```python
from build123d import *

# Parameters (mm, degrees)
F1_DEPTH = 40
F2_DEPTH = 5
F4_T     = -2
F3_R     = 35.75
F5_DEPTH = 5
F6_D     = 4.5
F6_DEPTH = 2
F6_TIP   = 1.3519363928
F8_DEPTH = 1.5


with BuildPart() as f1:
    # F0 (on Front) → F1 (new body, symmetric)
    with BuildSketch(Plane.XZ):
        Polygon((0, 69.2820323028), (-40, 0), (0, 0), align=None)
    extrude(amount=F1_DEPTH, both=True)

    # F2 (add): a face of the model
    f2_faces = [f1.faces().sort_by_distance(p)[0] for p in [
        (-20, 0, 34.6410161514),
    ]]
    extrude(f2_faces, amount=F2_DEPTH)

    # F4
    f4_openings = [f1.faces().sort_by_distance(p)[0] for p in [
        (-20, 0, 0),
    ]]
    offset(amount=F4_T, openings=f4_openings)

    # F3 (on face) → F5 (cut)
    with BuildSketch(Plane(origin=(-34.3301270189, 0, 19.8205080757), x_dir=(0, -1, 0), z_dir=(-0.8660254038, 0, 0.5))):
        with Locations((0, 20)):
            Circle(F3_R)
    extrude(amount=-F5_DEPTH, mode=Mode.SUBTRACT)

    # F6
    with Locations(Plane(origin=(-34.3301270189, 0, 19.8205080757), x_dir=(0, -1, 0), z_dir=(-0.8660254038, 0, 0.5))):
        with Locations((35.75, 55.75), (35.75, -15.75), (-35.75, -15.75), (-35.75, 55.75)):
            Hole(F6_D / 2, depth=F6_DEPTH)
            with Locations((0, 0, -(F6_DEPTH + F6_TIP / 2))):  # 118° drill point
                Cone(0, F6_D / 2, F6_TIP, mode=Mode.SUBTRACT)

    # F7 (on face) → F8 (cut)
    with BuildSketch(Plane(origin=(-32.5980762114, 0, 18.8205080757), x_dir=(0, 1, 0), z_dir=(0.8660254038, 0, -0.5))):
        Polygon((-33.7004065444, -12.2), (-37.7995934556, -12.2), (-39.8491869112, -15.75), (-37.7995934556, -19.3), (-33.7004065444, -19.3), (-31.6508130888, -15.75), align=None)
        Polygon((-37.7995934556, 55.3), (-39.8491869112, 51.75), (-37.7995934556, 48.2), (-33.7004065444, 48.2), (-31.6508130888, 51.75), (-33.7004065444, 55.3), align=None)
        Polygon((29.7004065444, -12.2), (27.6508130888, -15.75), (29.7004065444, -19.3), (33.7995934556, -19.3), (35.8491869112, -15.75), (33.7995934556, -12.2), align=None)
        Polygon((29.7004065444, 55.3), (27.6508130888, 51.75), (29.7004065444, 48.2), (33.7995934556, 48.2), (35.8491869112, 51.75), (33.7995934556, 55.3), align=None)
    extrude(amount=-F8_DEPTH, mode=Mode.SUBTRACT)

    # F9: F1 across face


with BuildPart() as f1_1:
    add(f1.part)
    add(f1.part.mirror(Plane(origin=(0, 0, 34.6410161514), x_dir=(0, 1, 0), z_dir=(1, 0, 0))))


solid = f1_1.part
```
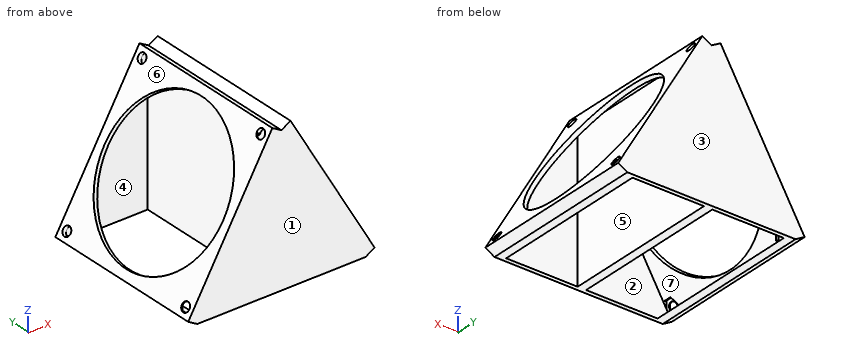
Work out the finished part from the listing and answer in its coordinate system (mm). Face numbers are marked on the shaded views. A direction names the side the tool comes from. Coordinates: 2 decimals unless noted, no trailing zeros. Write each loop counter-clockwise with the first axis right and the second up, starting at its lowest first coordinate (ties: lowest second). Pieces come first, ordered by that corner, then holes.
Q1. Which of the six approach directions +Z, -Z, +X, -X, +Y, -Y give full straight-line access (tool end or side, diameter ignored) to the marked faces 5, 6 and 7?
Q2. Each of these flat-tipped pins is pushed along its axis until it touches: pin 1 Ø1 at (y, z) = (-3, 8) entering from -X; pin 2 Ø6 at (y, z) = (-15.5, 31) entering from +X. Where does it stop, or does it pass through?
Q3. A cutting plane is placed at B-B, the plane y = -17. Give the vertices of the cut face in (x, z).
Q4. A cutting plane is placed at A-A, the plane y = 12. Give the vertices of the cut face in (x, z).
Q5. A cutting plane is placed at C-C, the plane y = 32. State how many separate pieces and enclosed holes the cut face has, then the cut area to 3 significant figures.
Q6. Determine the mould class of the marked faces 1, 2, 3 and 4 for opening direction Y: released by +Y, released by -Y, zero draft, split by the parting line, or undercut.
Q7. Find the intervals of material crossed by line 1 (Y direction, x = -13, z = 8.5); line 2 (X direction, y = 26.5, z = 15); line 3 (X direction, y = -17.5, z = 3.5), in increasing order.
Findings below:
1. face 5: -Z
1. face 6: +Z, -X, +Y, -Y
1. face 7: none
2. pin 1: stops at x = -2
2. pin 2: stops at x = 2
3. outline: (-44.33, 2.5) - (-40, 0) - (-36, 0) - (-41.6, 3.23) - (-38.32, 8.91) - (-40.05, 9.91) - close; (-8.61, 64.38) - (-6.87, 63.38) - (-3.6, 69.05) - (-2, 68.13) - (-2, 0) - (2, 0) - (2, 68.13) - (3.6, 69.05) - (6.87, 63.38) - (8.61, 64.38) - (4.33, 71.78) - (0, 69.28) - (-4.33, 71.78) - close; (36, 0) - (40, 0) - (44.33, 2.5) - (40.05, 9.91) - (38.32, 8.91) - (41.6, 3.23) - close
4. outline: (-44.33, 2.5) - (-40, 0) - (-36, 0) - (-41.6, 3.23) - (-39.44, 6.98) - (-41.17, 7.98) - close; (-7.49, 66.31) - (-5.76, 65.31) - (-3.6, 69.05) - (-2, 68.13) - (-2, 0) - (2, 0) - (2, 68.13) - (3.6, 69.05) - (5.76, 65.31) - (7.49, 66.31) - (4.33, 71.78) - (0, 69.28) - (-4.33, 71.78) - close; (36, 0) - (40, 0) - (44.33, 2.5) - (41.17, 7.98) - (39.44, 6.98) - (41.6, 3.23) - close
5. separate pieces: 3
5. enclosed holes: 0
5. area: 453 mm2
6. face 1: released by -Y
6. face 2: undercut
6. face 3: released by +Y
6. face 4: undercut
7. line 1: y = -40 to -38, 38 to 40
7. line 2: x = -37.11 to -34.8, -2 to 2, 34.8 to 37.11
7. line 3: x = -43.75 to -41.44, -2 to 2, 41.44 to 43.75
